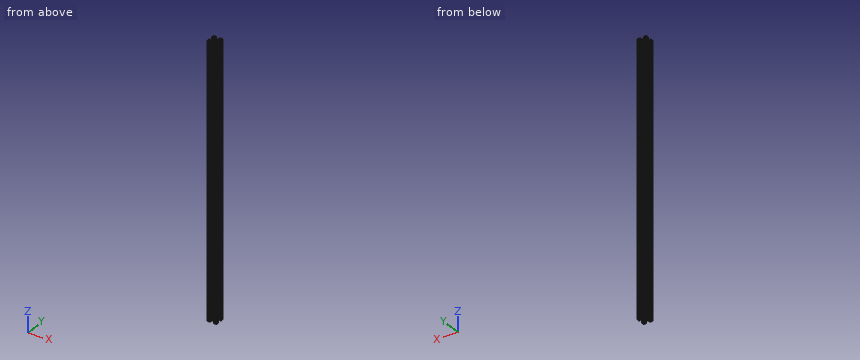
Autodesk Inventor part; units mm, degrees
ref_plane "Начальная плоскость" through (0, 0, 10) normal (0, 0, 1) x (1, 0, 0)
ref_plane "Конечная плоскость" through (0, 0, 600) normal (0, 0, 1) x (1, 0, 0)
ref_plane "РабПлоскость4" through (0, -300, 10) normal (0, 0, -1) x (-1, 0, 0)
ref_plane "Начальная плоскость" through (0, 0, 10) normal (0, 0, 1) x (1, 0, 0)
ref_plane "Конечная плоскость" through (0, 0, 600) normal (0, 0, 1) x (1, 0, 0)
sketch "Эскиз" plane through (0, 0, 0) normal (0, 0, 1) x (1, 0, 0)
  line L0 (-14.4349, 0) -> (14.4349, 0)
  line L1 (0, -14) -> (0, 14)
  line L2 (0, 0) -> (7.5, 7.5) construction
  circle A0 centre (7.5, 7.5) radius 1.65 construction
  line L3 (5.85, 9.15) -> (9.15, 9.15)
  line L4 (9.15, 9.15) -> (9.15, 5.85)
  line L5 (9.15, 5.85) -> (5.85, 5.85)
  line L6 (5.85, 5.85) -> (5.85, 9.15)
  line L7 (3.235, 8.1636) -> (4.72, 9.9636)
  line L8 (4.7971, 10) -> (8.5, 10)
  line L9 (3.3121, 8) -> (4.95, 8)
  line L10 (4.95, 8) -> (4.95, 5.7985)
  line L11 (4.95, 5.7985) -> (2.6515, 3.5)
  line L12 (0, 3.5) -> (2.6515, 3.5)
  circle A1 centre (0, 0) radius 2.5
  line L13 (8.1636, 3.235) -> (9.9636, 4.72)
  line L14 (10, 4.7971) -> (10, 8.5)
  line L15 (8, 3.3121) -> (8, 4.95)
  line L16 (8, 4.95) -> (5.7985, 4.95)
  line L17 (5.7985, 4.95) -> (3.5, 2.6515)
  line L18 (3.5, 0) -> (3.5, 2.6515)
  arc A2 (10, 8.5) -> (8.5, 10) centre (8.5, 8.5) ccw
  line L19 (0, 0) -> (-7.5, 7.5) construction
  circle A3 centre (-7.5, 7.5) radius 1.65 construction
  line L20 (-5.85, 9.15) -> (-9.15, 9.15)
  line L21 (-9.15, 9.15) -> (-9.15, 5.85)
  line L22 (-9.15, 5.85) -> (-5.85, 5.85)
  line L23 (-5.85, 5.85) -> (-5.85, 9.15)
  line L24 (-3.235, 8.1636) -> (-4.72, 9.9636)
  line L25 (-4.7971, 10) -> (-8.5, 10)
  line L26 (-3.3121, 8) -> (-4.95, 8)
  line L27 (-4.95, 8) -> (-4.95, 5.7985)
  line L28 (-4.95, 5.7985) -> (-2.6515, 3.5)
  line L29 (0, 3.5) -> (-2.6515, 3.5)
  line L30 (-3.5, 0) -> (-3.5, 2.6515)
  line L31 (-5.7985, 4.95) -> (-3.5, 2.6515)
  line L32 (-8, 4.95) -> (-5.7985, 4.95)
  line L33 (-8, 3.3121) -> (-8, 4.95)
  line L34 (-8.1636, 3.235) -> (-9.9636, 4.72)
  line L35 (-10, 4.7971) -> (-10, 8.5)
  arc A4 (-8.5, 10) -> (-10, 8.5) centre (-8.5, 8.5) ccw
  line L36 (0, 14) -> (0, -14)
  line L37 (0, 0) -> (7.5, -7.5) construction
  circle A5 centre (7.5, -7.5) radius 1.65 construction
  line L38 (5.85, -9.15) -> (9.15, -9.15)
  line L39 (9.15, -9.15) -> (9.15, -5.85)
  line L40 (9.15, -5.85) -> (5.85, -5.85)
  line L41 (5.85, -5.85) -> (5.85, -9.15)
  line L42 (3.235, -8.1636) -> (4.72, -9.9636)
  line L43 (4.7971, -10) -> (8.5, -10)
  line L44 (3.3121, -8) -> (4.95, -8)
  line L45 (4.95, -8) -> (4.95, -5.7985)
  line L46 (4.95, -5.7985) -> (2.6515, -3.5)
  line L47 (0, -3.5) -> (2.6515, -3.5)
  line L48 (3.5, 0) -> (3.5, -2.6515)
  line L49 (5.7985, -4.95) -> (3.5, -2.6515)
  line L50 (8, -4.95) -> (5.7985, -4.95)
  line L51 (8, -3.3121) -> (8, -4.95)
  line L52 (8.1636, -3.235) -> (9.9636, -4.72)
  line L53 (10, -4.7971) -> (10, -8.5)
  arc A6 (8.5, -10) -> (10, -8.5) centre (8.5, -8.5) ccw
  line L54 (0, 0) -> (-7.5, -7.5) construction
  line L55 (-4.95, -8) -> (-4.95, -5.7985)
  line L56 (-3.3121, -8) -> (-4.95, -8)
  line L57 (-5.7985, -4.95) -> (-3.5, -2.6515)
  line L58 (-4.95, -5.7985) -> (-2.6515, -3.5)
  line L59 (-3.5, 0) -> (-3.5, -2.6515)
  line L60 (0, -3.5) -> (-2.6515, -3.5)
  circle A7 centre (-7.5, -7.5) radius 1.65 construction
  line L61 (-5.85, -5.85) -> (-5.85, -9.15)
  line L62 (-5.85, -9.15) -> (-9.15, -9.15)
  line L63 (-9.15, -9.15) -> (-9.15, -5.85)
  line L64 (-9.15, -5.85) -> (-5.85, -5.85)
  line L65 (-3.235, -8.1636) -> (-4.72, -9.9636)
  line L66 (-8, -4.95) -> (-5.7985, -4.95)
  line L67 (-8, -3.3121) -> (-8, -4.95)
  line L68 (-8.1636, -3.235) -> (-9.9636, -4.72)
  line L69 (-4.7971, -10) -> (-8.5, -10)
  line L70 (-10, -4.7971) -> (-10, -8.5)
  arc A8 (-10, -8.5) -> (-8.5, -10) centre (-8.5, -8.5) ccw
  arc A9 (3.235, 8.1636) -> (3.3121, 8) centre (3.3121, 8.1) ccw
  arc A10 (4.7971, 10) -> (4.72, 9.9636) centre (4.7971, 9.9) ccw
  arc A11 (8, 3.3121) -> (8.1636, 3.235) centre (8.1, 3.3121) ccw
  arc A12 (9.9636, 4.72) -> (10, 4.7971) centre (9.9, 4.7971) ccw
  arc A13 (-3.3121, 8) -> (-3.235, 8.1636) centre (-3.3121, 8.1) ccw
  arc A14 (-4.72, 9.9636) -> (-4.7971, 10) centre (-4.7971, 9.9) ccw
  arc A15 (-8.1636, 3.235) -> (-8, 3.3121) centre (-8.1, 3.3121) ccw
  arc A16 (-10, 4.7971) -> (-9.9636, 4.72) centre (-9.9, 4.7971) ccw
  arc A17 (-8, -3.3121) -> (-8.1636, -3.235) centre (-8.1, -3.3121) ccw
  arc A18 (-9.9636, -4.72) -> (-10, -4.7971) centre (-9.9, -4.7971) ccw
  arc A19 (-3.235, -8.1636) -> (-3.3121, -8) centre (-3.3121, -8.1) ccw
  arc A20 (-4.7971, -10) -> (-4.72, -9.9636) centre (-4.7971, -9.9) ccw
  arc A21 (4.72, -9.9636) -> (4.7971, -10) centre (4.7971, -9.9) ccw
  arc A22 (3.3121, -8) -> (3.235, -8.1636) centre (3.3121, -8.1) ccw
  arc A23 (8.1636, -3.235) -> (8, -3.3121) centre (8.1, -3.3121) ccw
  arc A24 (10, -4.7971) -> (9.9636, -4.72) centre (9.9, -4.7971) ccw
  point P0 (3.1, 8)
  point P1 (4.75, 10)
  point P2 (7.5, 9.15)
  point P3 (8, 3.1)
  point P4 (10, 4.75)
  point P5 (7.5, 5.85)
  point P6 (9.15, 7.5)
  point P7 (-3.1, 8)
  point P8 (-4.75, 10)
  point P9 (-7.5, 9.15)
  point P10 (-8, 3.1)
  point P11 (-10, 4.75)
  point P12 (-7.5, 5.85)
  point P13 (-9.15, 7.5)
  point P14 (3.1, -8)
  point P15 (4.75, -10)
  point P16 (7.5, -9.15)
  point P17 (8, -3.1)
  point P18 (10, -4.75)
  point P19 (7.5, -5.85)
  point P20 (9.15, -7.5)
  point P21 (-3.1, -8)
  point P22 (-7.5, -5.85)
  point P23 (-7.5, -9.15)
  point P24 (-9.15, -7.5)
  point P25 (-4.75, -10)
  point P26 (-8, -3.1)
  point P27 (-10, -4.75)
  dimension "d0" = 45
  dimension "d1" = 3.3
  dimension "d2" = 1.5
  dimension "d3" = 1.2
  dimension "d4" = 5
  dimension "d5" = 6.5
  dimension "d6" = 15
  dimension "d7" = 20
  dimension "d8" = 9.9
  dimension "d9" = 9.5
  dimension "d10" = 6.2
  dimension "d11" = 2
  dimension "d18" = 0.1
  dimension "d19" = 0.1
extrude "Тело" add sketch "Эскиз" along normal up to surface (590 mm away) from surface at 10 contours A1 L1 L12 L11 L10 L9 A9 L7 A10 L8 A2 L14 A12 L13 A11 L15 L16 L17 L18 L0 | L0 L48 L49 L50 L51 A23 L52 A24 L53 A6 L43 A21 L42 A22 L44 L45 L46 L47 L1 A1 | A1 L0 L30 L31 L32 L33 A15 L34 A16 L35 A4 L25 A14 L24 A13 L26 L27 L28 L29 L1 | L1 L60 L58 L55 L56 A19 L65 A20 L69 A8 L70 A18 L68 A17 L67 L66 L57 L59 L0 A1
sketch "Эскиз2" plane through (0, 0, 0) normal (0, 0, 1) x (1, 0, 0)
  line L0 (0, 0) -> (10, 0)
ref_plane "РабПлоскость3" through (0, 0, 0) normal (0, -1, 0) x (1, 0, 0)
sketch "Эскиз3" plane through (0, 0, 0) normal (0, -1, 0) x (1, 0, 0)
  line L0 (-2, 10) -> (12, 10)
  line L1 (-2, 600) -> (12, 600)
  dimension "d25" = 590
ref_plane "РабПлоскость4" through (0, -300, 10) normal (0, 0, -1) x (-1, 0, 0)
split "Разделение1" plane through (0, -300, 10) removes the side toward (0, 0, -1)
ref_plane "РабПлоскость5" through (50, 0, 10) normal (0, 0, -1) x (-1, 0, 0)
split "Разделение2" plane through (50, 0, 10) removes the side toward (0, 0, -1)
equation "\"G_OFFSET_END\" = 0"
properties part number "короткая палка"
CAD build for the part. Positions are in the model's coordinates, mm. Round coordinates to 2 decimals unless told otherwise and drop trailing zeros.
(1) Drop flat-ended pins along their axis: pin 1 (1.5 mm diameter, centred on y = -1, z = 179, fed in from -X); pin 2 (4 mm diameter, centred on x = -1.5, z = 266.5, fed in from -Y); pin 3 (1 mm diameter, centred on y = 4, z = 353.5, fed in from +X); pin 4 (3 mm diameter, centred on x = -8, y = 0, fed in from -Z). Give the stop position or say it passes through.
(2) Cut at A-A (z = 494). State how many separate pieces and enclosed holes the cut face has, plus the area to 3 significant figures.
(3) Wall check: line 1 along Y through (x, z) = (8.25, 314); line 2 along X through (y, z) = (-7.75, 122.5); line 3 along X through (y, z) = (0, 265). Give the ranges that are in metal, low to high.
Findings below:
1. pin 1: stops at x = -3.5
1. pin 2: stops at y = -8.48
1. pin 3: stops at x = 9.7
1. pin 4: passes through
2. separate pieces: 1
2. enclosed holes: 5
2. area: 115 mm2
3. line 1: y = -10 to -9.15, -5.85 to -3.31, 3.31 to 5.85, 9.15 to 10
3. line 2: x = -10 to -9.15, -5.85 to -4.95, 4.95 to 5.85, 9.15 to 10
3. line 3: x = -3.5 to -2.5, 2.5 to 3.5
